```python
from build123d import *

# Parameters (mm, degrees)
F5_R      = 101.6
F4_R      = 127
F7_R      = 76.2
F8_DEPTH  = 304.8
F9_R      = 75.7174
F10_DEPTH = 304.8
F11_R     = 126.5174
F12_R     = 101.1174


with BuildPart() as f6:
    # F5 (on face) → F6 section 0
    with BuildSketch(Plane(origin=(0, 0, 508), x_dir=(1, 0, 0), z_dir=(0, 0, -1))):
        Circle(F5_R)
    # F4 (on face) → F6 section 1
    with BuildSketch(Plane.XY):
        Circle(F4_R)
    loft()

    # F7 (on face) → F8 (join)
    with BuildSketch(Plane(origin=(327.647171, 0, 327.647171), x_dir=(0.707107, 0, -0.707107), z_dir=(0.707107, 0, 0.707107))):
        with Locations((-107.763073, 0)):
            Circle(F7_R)
    extrude(amount=-F8_DEPTH)

    # F9 (on face) → F10 (cut)
    with BuildSketch(Plane(origin=(327.647171, 0, 327.647171), x_dir=(0.707107, 0, -0.707107), z_dir=(0.707107, 0, 0.707107))):
        with Locations((-107.763073, 0)):
            Circle(F9_R)
    extrude(amount=-F10_DEPTH, mode=Mode.SUBTRACT)

    # F11 (on face) → F13 section 0
    with BuildSketch(Plane(origin=(0, 0, 0), x_dir=(1, 0, 0), z_dir=(0, 0, -1))):
        Circle(F11_R)
    # F12 (on face) → F13 section 1
    with BuildSketch(Plane.XY.offset(508)):
        Circle(F12_R)
    loft(mode=Mode.SUBTRACT)


solid = f6.part
```
Read the model definition and answer for the solid it produces. Units are mm, in the model's axes. Coordinates: 2 decimals unless noted, no trailing zeros. Loops run counter-clockwise (first coordinate to the right, second up) from the corner with the lowest first, then second, coordinate; pieces in that order, holes last. Notation, with made-up numbers: (18, -15.5) - (35, -15.5) arc R12 cw to (35, 6.5) - close; hole circle Ø4 at (22, -30.75). An arc over 180 degrees is marked (long way). Answer in a Markdown table with one row per item.
1. Given pin 1 (5 mm diameter, centred on x = -29.5, z = 333, fed in from -Y); pin 2 (8 mm diameter, centred on y = 74, z = 60, fed in from +X); pin 3 (10 mm diameter, centred on y = -5, z = 195.5, fed in from -X), each flat-ended and moving along its own axis, determine where each tip first touches the part or whether it passes through.
Conclusion:
| item | result |
|---|---|
| pin 1 | stops at y = -107.01 |
| pin 2 | stops at x = 102.36 |
| pin 3 | stops at x = -117.42 |
2. Find section B-B, the plane y = -57.5. Count the separate pieces of the cut face and the enclosed holes in it, then the cut area to 3 significant figures.
Conclusion:
| item | result |
|---|---|
| separate pieces | 3 |
| enclosed holes | 0 |
| area | 814 mm² |
3. Find section A-A, the plane x = 0. Write down the section's boundary in (y, z), then the cut area to 3 significant figures.
Conclusion:
| item | result |
|---|---|
| outline | (-127, 0) - (-126.52, 0) - (-101.12, 508) - (-101.6, 508) - close; (101.12, 508) - (126.52, 0) - (127, 0) - (101.6, 508) - close |
| area | 490 mm² |
4. Determine the mould class of faces 1 (the face through (231.234, 22.743, 281.499)), 2 (the face through (-113.53, -5, 257.56)) for opening direction Z: +Z half, -Z half, draft (parallel to the pull), parting line (faces both ways), or undercut.
Conclusion:
| item | result |
|---|---|
| face 1 | undercut |
| face 2 | -Z half |
5. Find section C-C, the plane z = 140. Write down the section's boundary in (x, y).
Conclusion:
| item | result |
|---|---|
| outline | circle Ø240 at (0, 0); hole circle Ø239.03 at (0, 0) |
